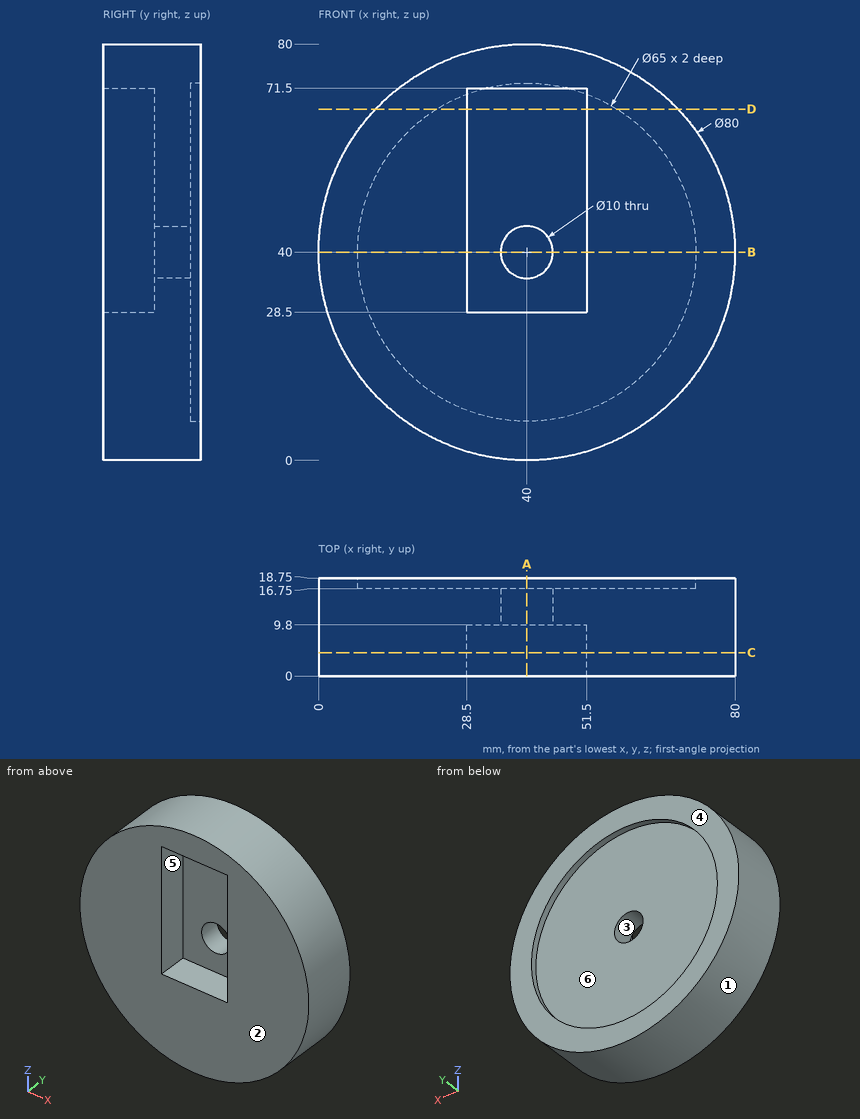
Check sheet for the drawn part. Datum: minimum x, y, z corner. Units: mm. A direction names the side the tool comes from. Coordinates: 2 decimals unless noted, no trailing zeros. Loops run counter-clockwise (first coordinate to the right, second up) from the corner with the lowest first, then second, coordinate; pieces in that order, holes last. Notation, with made-up numbers: (82, 16) - (137, 16) arc R25 cw to (137, 52) - close; hole circle Ø11 at (-16, 22). An arc over 180 degrees is marked (long way). Put each result on its own line as item: value.
Item 1: Scan lines: line 1 along X through (y, z) = (14, 40); line 2 along X through (y, z) = (17.55, 40); line 3 along Y through (x, z) = (25, 55). Record each from-to range of solid material in increasing order.
Conclusion:
line 1: x = 0 to 35, 45 to 80
line 2: x = 0 to 7.5, 72.5 to 80
line 3: y = 0 to 16.75
Item 2: Section check A-A (x = 40). Enter the section's corners in (y, z).
Conclusion:
outline: (0, 0) - (18.75, 0) - (18.75, 7.5) - (16.75, 7.5) - (16.75, 35) - (9.8, 35) - (9.8, 28.5) - (0, 28.5) - close; (0, 71.5) - (9.8, 71.5) - (9.8, 45) - (16.75, 45) - (16.75, 72.5) - (18.75, 72.5) - (18.75, 80) - (0, 80) - close
Item 3: Section check D-D (z = 67.5). Enter the section's corners in (x, y), then the cut area to 3 significant figures.
Conclusion:
outline: (10.95, 0) - (28.5, 0) - (28.5, 9.8) - (51.5, 9.8) - (51.5, 0) - (69.05, 0) - (69.05, 18.75) - (57.32, 18.75) - (57.32, 16.75) - (22.68, 16.75) - (22.68, 18.75) - (10.95, 18.75) - close
area: 795 mm2
Item 4: Section check C-C (y = 4.5). Enter the section's corners in (x, z), then the cut area to 3 significant figures.
Conclusion:
outline: circle Ø80 at (40, 40); hole (28.5, 28.5) - (51.5, 28.5) - (51.5, 71.5) - (28.5, 71.5) - close
area: 4,040 mm2
Item 5: Draft check along Z on the marked faces 1, 2 and 3. Enter one of: pulls with the +Z half, pulls with the -Z half, needs draft (parallel to the pull), parting line crosses it, or undercut.
Conclusion:
face 1: parting line crosses it
face 2: needs draft
face 3: undercut
Item 6: Gauge pin test, flat ends, axial feed: pin 1 Ø11 at (y, z) = (3, 46) entering from +X; pin 2 Ø10 at (x, y) = (23, 13) entering from -Z; pin 3 Ø2 at (y, z) = (8.5, 52.5) entering from -X. Record the tip position at first contact, or that the pin passes through.
Conclusion:
pin 1: stops at x = 80
pin 2: stops at z = 1.84
pin 3: stops at x = 1.69
Item 7: Section check B-B (z = 40). Enter the section's corners in (x, y).
Conclusion:
outline: (0, 0) - (28.5, 0) - (28.5, 9.8) - (35, 9.8) - (35, 16.75) - (7.5, 16.75) - (7.5, 18.75) - (0, 18.75) - close; (45, 9.8) - (51.5, 9.8) - (51.5, 0) - (80, 0) - (80, 18.75) - (72.5, 18.75) - (72.5, 16.75) - (45, 16.75) - close
Item 8: Set-up check for the marked faces 4, 5 and 6: record each of +Z, -Z, +X, -X, +Y, -Y from which the full face is reachable in a straight line by a thin tool's end or side.
Conclusion:
face 4: +Z, -Z, +X, -X, +Y
face 5: -Y
face 6: +Y
